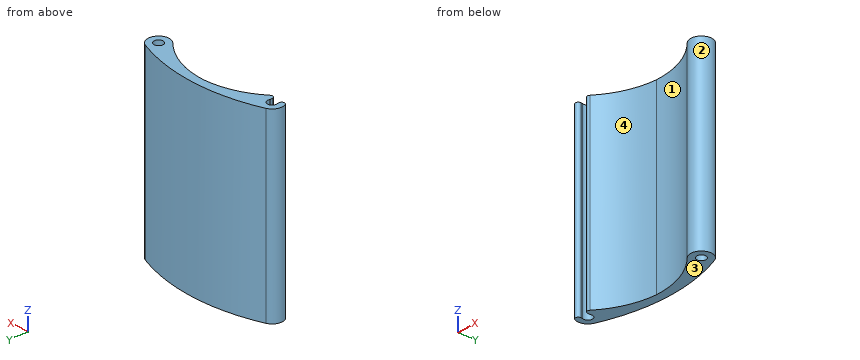
Autodesk Inventor part; units mm, degrees
ref_plane "YZ Plane" through (0, 0, 0) normal (1, 0, 0) x (0, 1, 0)
ref_plane "XZ Plane" through (0, 0, 0) normal (0, 1, 0) x (-1, 0, 0)
ref_plane "XY Plane" through (0, 0, 0) normal (0, 0, 1) x (1, 0, 0)
ref_plane "作業平面1" through (0, 0, 0) normal (0, 0, 1) x (1, 0, 0)
sketch "スケッチ1" plane through (0, 0, 0) normal (0, 0, 1) x (1, 0, 0)
  circle A0 centre (250, 230) radius 3 construction
  line L0 (246.124, 222.5) -> (255, 222.5) construction
  circle A1 centre (239, 219) radius 3 construction
  circle A2 centre (161.1336, 230) radius 3 construction
  arc A3 (-159.3342, 234.665) -> (159.3342, 234.665) centre (0, 647.734) ccw construction
  line L1 (250, 235) -> (161.1336, 235) construction
  circle A4 centre (250, 230) radius 3.2
  circle A5 centre (161.1336, 230) radius 3.2
  circle A6 centre (250, 230) radius 7.5 construction
  circle A7 centre (161.1336, 230) radius 7.5 construction
  line L2 (250, 230) -> (161.1336, 230) construction
  line L3 (205.5668, 230) -> (205.5668, 246) construction
  arc A8 (252.7682, 236.9705) -> (158.3654, 236.9705) centre (205.5668, 118.1142) ccw
  arc A9 (243.602, 233.9135) -> (167.5316, 233.9135) centre (205.5668, 118.1142) ccw
  arc A10 (243.602, 233.9135) -> (252.7682, 236.9705) centre (250, 230) ccw
  arc A11 (158.3654, 236.9705) -> (167.5316, 233.9135) centre (161.1336, 230) ccw
  point P0 (0, 0)
  dimension "d0" = 6.4
  dimension "d1" = 15
  dimension "d2" = 16
  dimension "d3" = 6
extrude "押し出し1" add sketch "スケッチ1" along normal blind 130
fillet "フィレット1" radius 60 2 edges at (243.602, 233.9135, 65) (167.5316, 233.9135, 65)
sketch "スケッチ2" plane through (0, 0, 0) normal (0, 0, -1) x (-1, 0, 0)
  arc A0 (-166.1782, 224.45) -> (-158.3654, 236.9705) centre (-161.1336, 230) ccw
  circle A1 centre (-161.1336, 230) radius 3.2
  circle A2 centre (-250, 230) radius 3.2
  circle A3 centre (-250, 230) radius 88.8664 construction
  arc A4 (-158.4511, 222.9961) -> (-158.1923, 228.7397) centre (-250, 230) ccw
  arc A5 (-164.3511, 223.2252) -> (-164.0923, 228.7808) centre (-250, 230) ccw
  point P0 (0, 0)
  dimension "d7" = 2.95
  dimension "d8" = 2.95
extrude "押し出し2" cut sketch "スケッチ2" against normal through all contours A5 A1 A4 A0
fillet "フィレット2" radius 2 4 edges at (158.4511, 222.9961, 65) (164.3511, 223.2252, 65) (164.0923, 228.7808, 65) (158.1923, 228.7397, 65)
equation "\"d8\" = d7"
properties part number "foot_01"
Part model, mm, in its own coordinate system. Face numbers are marked on the shaded views. Give positions to 0.01 mm unless a question says otherwise; leave off trailing zeros. Order: outer loops, then holes, each group sorted by start corner. A loop starts at its lowest first (then second) coordinate and runs counter-clockwise, first axis right, second up. Notation, with made-up numbers: M 85,12.25 L 127,12.25 A28 ccw 127,50.25 Z; hole C 45.25,24 d4. An arc over 180 degrees is marked long. Use a Markdown table: item, result. Add a question column.
(1) Saw through at A-A, the plane y = 235.5. Give the cut face in (x, z), and give its area (3 significant figures).
(2) Drop flat-ended pins along their axis: P1, Ø4, axis at x = 161.13, y = 230, coming from the +Z side; P2, Ø2, axis at y = 235, z = 17.5, coming from the +X side; P3, Ø2, axis at y = 234, z = 96, coming from the +X side; P4, Ø2, axis at x = 214.5, z = 101.5, coming from the -Y side. Give the stop position or say it passes through.
(3) Saw through at D-D, the plane y = 244. Give the cut face in (x, z), and give its area (3 significant figures).
(4) Saw through at C-C, the plane x = 215. Give the cut face in (y, z).
(5) Saw through at B-B, the plane x = 250. Give the cut face in (y, z).
(6) Mould opens along X. For the marked faces 1, 2, 3 and 4 say: +X half, -X half, draft (parallel to the pull), parting line (faces both ways), or undercut.
(7) Probe line 1 along X through (y, z) = (230, 15.5); line 2 along X through (y, z) = (229.75, 111.5); line 3 along Y through (x, z) = (206.5, 7). List the from-to ranges inside material, lowest first. Write a range as [from, to].
Answer key:
| question | item | result |
|---|---|---|
| 1 | outline | M 156.03,0 L 183.62,0 L 183.62,130 L 156.03,130 Z; M 227.44,0 L 255.1,0 L 255.1,130 L 227.44,130 Z |
| 1 | area | 7,180 mm^2 |
| 2 | P1 | through |
| 2 | P2 | x = 256.34 |
| 2 | P3 | x = 256.87 |
| 2 | P4 | y = 239.01 |
| 3 | outline | M 183.04,0 L 228.1,0 L 228.1,130 L 183.04,130 Z |
| 3 | area | 5,860 mm^2 |
| 4 | outline | M 239.1,0 L 245.65,0 L 245.65,130 L 239.1,130 Z |
| 5 | outline | M 222.5,0 L 226.8,0 L 226.8,130 L 222.5,130 Z; M 233.2,0 L 238.03,0 L 238.03,130 L 233.2,130 Z |
| 6 | face 1 | undercut |
| 6 | face 2 | parting line |
| 6 | face 3 | draft |
| 6 | face 4 | undercut |
| 7 | line 1 | [153.63, 157.93], [164.33, 173.29], [237.82, 246.8], [253.2, 257.5] |
| 7 | line 2 | [153.64, 157.94], [164.32, 172.92], [238.19, 246.81], [253.19, 257.5] |
| 7 | line 3 | [239.97, 246] |
